```python
from build123d import *

# Parameters (mm, degrees)
EXTRUDE_1_DEPTH      = 8
SKETCH_2_W           = 9
SKETCH_2_H           = 8
EXTRUDE_2_DEPTH      = 3
SKETCH_3_OUTSIDE_W   = 15.256
SKETCH_3_OUTSIDE_H   = 13.318
SKETCH_3_OUTSIDE_W_2 = 5.2
SKETCH_3_OUTSIDE_H_2 = 7
SKETCH_3_OUTSIDE_W_3 = 2
SKETCH_3_OUTSIDE_H_3 = 5
CUT_EXTRUDE_1_DEPTH  = 3.5
EXTRUDE_3_DEPTH      = 1


with BuildPart() as part:
    # 草图1 → 凸台-拉伸1 (new body)
    with BuildSketch(Plane.XY):
        Polygon((-3.062050808, 3.303627574), (-4.969401077, 0), (-2.484700538, -4.303627574), (2.484700538, -4.303627574), (4.969401077, 0), (3.062050808, 3.303627574), (1.33, 2.303627574), (2.66, 0), (1.33, -2.303627574), (-1.33, -2.303627574), (-2.66, 0), (-1.33, 2.303627574), align=None)
    extrude(amount=EXTRUDE_1_DEPTH)

    # 草图2 → 凸台-拉伸2 (add)
    with BuildSketch(Plane.XZ.offset(4.303627574)):
        with Locations((0, 4)):
            Rectangle(SKETCH_2_W, SKETCH_2_H)
    extrude(amount=EXTRUDE_2_DEPTH)

    # 草图3 outside → 切除-拉伸1 (cut)
    # profile 1 of 2: a face of its own
    with BuildSketch(Plane.XZ.offset(7.303627574)):
        with Locations((0, 4)):
            Rectangle(SKETCH_3_OUTSIDE_W, SKETCH_3_OUTSIDE_H)
        with Locations((0, 4)):
            Rectangle(SKETCH_3_OUTSIDE_W_2, SKETCH_3_OUTSIDE_H_2, mode=Mode.SUBTRACT)
    # profile 2 of 2: a face of its own
    with BuildSketch(Plane.XZ.offset(7.303627574)):
        with Locations((0, 4)):
            Rectangle(SKETCH_3_OUTSIDE_W_3, SKETCH_3_OUTSIDE_H_3)
    extrude(amount=-CUT_EXTRUDE_1_DEPTH, mode=Mode.SUBTRACT)

    # 草图4 → 凸台-拉伸3 (add)
    with BuildSketch(Plane.XY.offset(8)):
        Polygon((-4.276580754, 0), (-2.426965511, -3.203627574), (2.426965511, -3.203627574), (4.276580754, 0), (2.842435565, 2.484012332), (2.149615242, 2.084012332), (3.352820323, 0), (1.676410162, -2.903627574), (-1.676410162, -2.903627574), (-3.352820323, 0), (-2.149615242, 2.084012332), (-2.842435565, 2.484012332), align=None)
    extrude(amount=EXTRUDE_3_DEPTH)


solid = part.part
```
Source: CAD feature listing. Evaluate the final solid. Frame: model axes, mm. A direction names the side the tool comes from. Round coordinates to 2 decimals unless told otherwise and drop trailing zeros. Order: outer loops, then holes, each group sorted by start corner. A loop starts at its lowest first (then second) coordinate and runs counter-clockwise, first axis right, second up. Notation, with made-up numbers: (47, -27.5) -> (94, -27.5) arc R26 ccw to (94, -7.5) -> close; hole circle Ø6 at (-20, 1). An arc over 180 degrees is marked (long way). One line per item, written item: value. Start each with the question number.
Q1. Draft query along Z for faces 6 (the flat face through (0, -3.804, 4)), 7 (the flat face through (-2.76, 1.03, 8.49)). Return one class per face: pulls with the +Z half, pulls with the -Z half, needs draft (parallel to the pull), parting line crosses it, or undercut.
Q2. Pin query (flat end, axial travel): pin 1 (0.9 mm diameter, centred on y = -6, z = 2.5, fed in from -X); pin 2 (1.8 mm diameter, centred on x = -0.5, y = -5.5, fed in from +Z); pin 3 (1.8 mm diameter, centred on y = -6, z = 3, fed in from +X); pin 4 (2 mm diameter, centred on x = 2.5, y = 2, fed in from -Z). Return the tip coordinate at first contact, or that it passes through.
Q3. Section query A-A (y = 1.5). Return the cut outline in (x, z).
Q4. Access query for faces 1 (the flat face through (-2.6, -6, 4)), 2 (the flat face through (0, -3.204, 8.5)), 3 (the flat face through (-2.503, -1.472, 8.493)), 4 (the flat face through (3.57, 1.22, 8.49)), 5 (the flat face through (2.6, -6, 4)). Directions: +Z, -Z, +X, -X, +Y, -Y. A direction counts if a zero-diameter tool reaches every point of the face in a straight line with its end or side. Return the directions, or none.
Q5. Section query B-B (x = 1.5). Return the cut outline in (y, z), plus the area to 3 significant figures.
Q6. Section query D-D (y = -5.5). Return the cut outline in (x, z).
Q7. Section query C-C (x = 0.5). Return the cut outline in (y, z), plus the area to 3 significant figures.
Q8. Material intervals for probe 1 along Z at (x, y) = (-0.5, -5.5); probe 2 along X at (y, z) = (-6.5, 4); probe 3 along Y at (x, z) = (0, 1.25), sorted ascending.
Findings below:
1. face 6: undercut
1. face 7: needs draft
2. pin 1: x = -2.6
2. pin 2: z = 7.5
2. pin 3: x = 2.6
2. pin 4: z = 0
3. outline: (-4.1, 0) -> (-1.79, 0) -> (-1.79, 8) -> (-2.49, 8) -> (-2.49, 9) -> (-3.41, 9) -> (-3.41, 8) -> (-4.1, 8) -> close; (1.79, 0) -> (4.1, 0) -> (4.1, 8) -> (3.41, 8) -> (3.41, 9) -> (2.49, 9) -> (2.49, 8) -> (1.79, 8) -> close
4. face 1: +Z, -Z, -X, -Y
4. face 2: +Z, +X, -X, -Y
4. face 3: +Z
4. face 4: +Z, +X, +Y
4. face 5: +Z, -Z, +X, -Y
5. outline: (-7.3, 0.5) -> (-3.8, 0.5) -> (-3.8, 0) -> (-2.01, 0) -> (-2.01, 8) -> (-2.9, 8) -> (-2.9, 9) -> (-3.2, 9) -> (-3.2, 8) -> (-3.8, 8) -> (-3.8, 7.5) -> (-7.3, 7.5) -> close; (2.01, 0) -> (2.4, 0) -> (2.4, 8) -> (2.01, 8) -> close
5. area: 42.3 mm²
6. outline: (-2.6, 0.5) -> (2.6, 0.5) -> (2.6, 7.5) -> (-2.6, 7.5) -> close; hole (-1, 1.5) -> (1, 1.5) -> (1, 6.5) -> (-1, 6.5) -> close
7. outline: (-7.3, 0.5) -> (-3.8, 0.5) -> (-3.8, 0) -> (-2.3, 0) -> (-2.3, 8) -> (-2.9, 8) -> (-2.9, 9) -> (-3.2, 9) -> (-3.2, 8) -> (-3.8, 8) -> (-3.8, 7.5) -> (-7.3, 7.5) -> (-7.3, 6.5) -> (-3.8, 6.5) -> (-3.8, 1.5) -> (-7.3, 1.5) -> close
7. area: 19.3 mm²
8. probe 1: 0.5 to 1.5, 6.5 to 7.5
8. probe 2: -2.6 to -1, 1 to 2.6
8. probe 3: -7.3 to -2.3
